Input: dimensioned drawing with shaded views. Units: mm. Origin: part minimum x, y, z. Give positions to 0.01 mm unless a question says otherwise; leave off trailing zeros. Loops run counter-clockwise (first coordinate to the right, second up) from the corner with the lowest first, then second, coordinate; pieces in that order, holes last. Notation, with made-up numbers: M 17,-40 L 71,-40 A17 ccw 71,-25 Z; hole C 85.5,60 d9. An arc over 180 degrees is marked long. One line per question, with ' | ' between items. Start each with the question number.
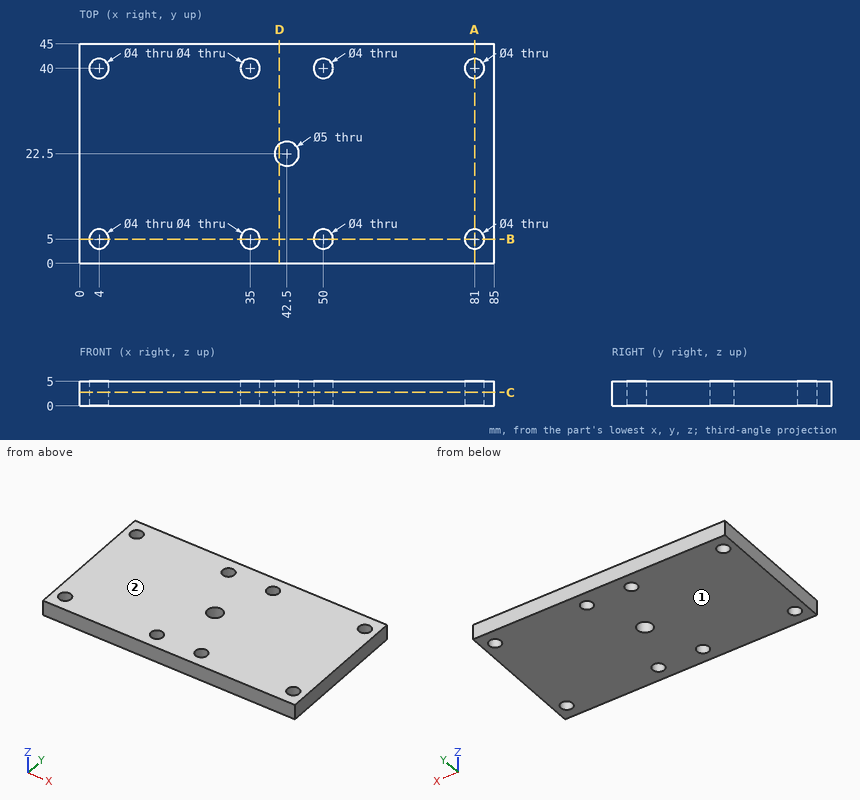
Q1. Section D-D, the plane x = 41. Output: boundary loops of the cut face in (y, z).
Q2. Material intervals for L1, parallel to Y at x = 81, z = 2.3; L2, parallel to X at y = 4, z = 4.05; L3, parallel to X at y = 3.5, z = 3.9, sorted ascending.
Q3. Section A-A, the plane x = 81. Output: boundary loops of the cut face in (y, z), plus the area to 3 significant figures.
Q4. Section C-C, the plane z = 2.75. Count the separate pieces of the cut face and the enclosed holes in it, plus the area to 3 significant figures.
Q5. Contact query for a flat-ended pin moving along its axis: pin 1 (2.5 mm diameter, centred on x = 81, y = 5, fed in from -Z). Output: stop coordinate, or through.
Q6. Draft query along Z for the marked faces 1 and 2. Return one class per face: released by +Z, released by -Z, zero draft, split by the parting line, or undercut.
Q7. Section B-B, the plane y = 5. Output: boundary loops of the cut face in (x, z).
Model answer:
1) outline: M 0,0 L 20.5,0 L 20.5,5 L 0,5 Z; M 24.5,0 L 45,0 L 45,5 L 24.5,5 Z
2) L1: y = 0 to 3, 7 to 38, 42 to 45 | L2: x = 0 to 2.27, 5.73 to 33.27, 36.73 to 48.27, 51.73 to 79.27, 82.73 to 85 | L3: x = 0 to 2.68, 5.32 to 33.68, 36.32 to 48.68, 51.32 to 79.68, 82.32 to 85
3) outline: M 0,0 L 3,0 L 3,5 L 0,5 Z; M 7,0 L 38,0 L 38,5 L 7,5 Z; M 42,0 L 45,0 L 45,5 L 42,5 Z | area: 185 mm^2
4) separate pieces: 1 | enclosed holes: 9 | area: 3,700 mm^2
5) pin 1: passes through
6) face 1: released by -Z | face 2: released by +Z
7) outline: M 0,0 L 2,0 L 2,5 L 0,5 Z; M 6,0 L 33,0 L 33,5 L 6,5 Z; M 37,0 L 48,0 L 48,5 L 37,5 Z; M 52,0 L 79,0 L 79,5 L 52,5 Z; M 83,0 L 85,0 L 85,5 L 83,5 Z
